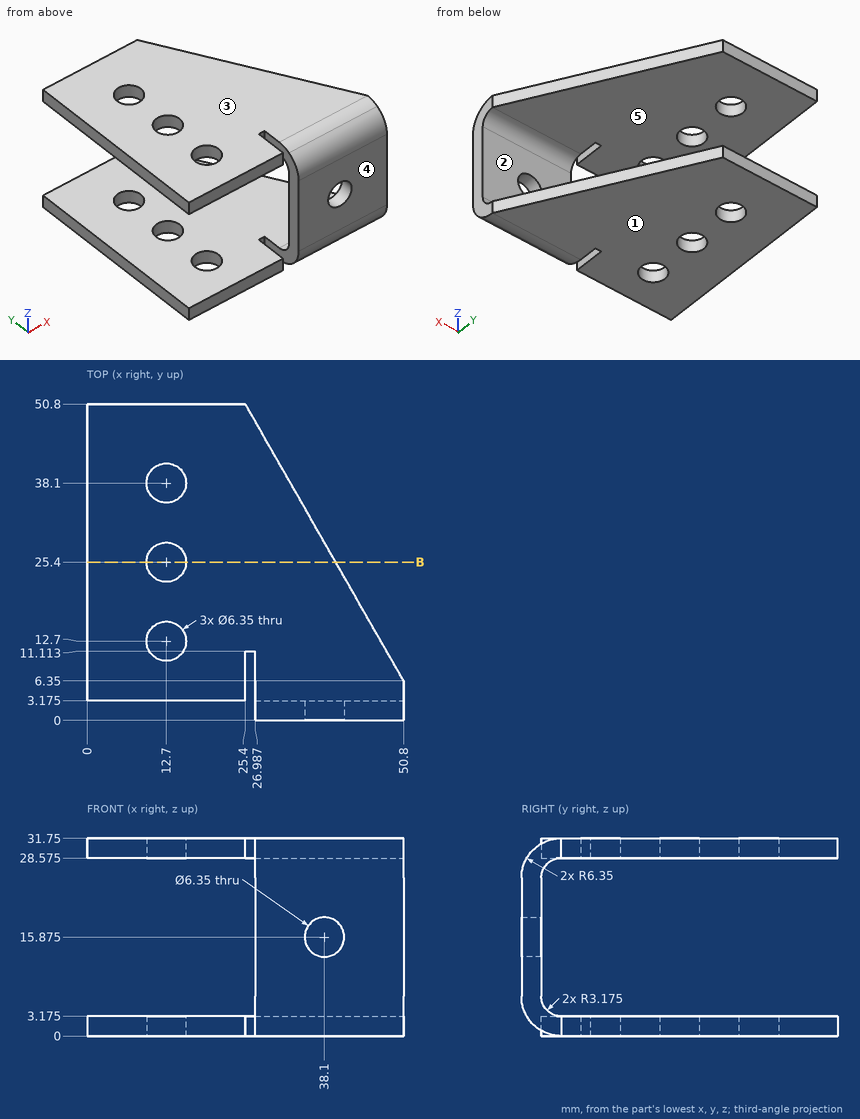
For this review, use the dimensioned drawing (mm, ordinates from the lowest corner) and the shaded views. A direction names the side the tool comes from. Coordinates: 2 decimals unless noted, no trailing zeros. Use a Markdown table: item, result. Add a question column.
Item 1: We need section B-B, the plane y = 25.4. Count the separate pieces of the cut face and the enclosed holes in it, and give its area (3 significant figures).
Item 2: Wall thickness on L1, parallel to Y at x = 12.7, z = 2.5 (1 decimal); L2, parallel to Y at x = 16, z = 3 (1 decimal); L3, parallel to Y at x = 12, z = 1 (1 decimal): over which ranges is each line inside the solid? List them lowest first. Write a range as from..to.
Item 3: Clearance check with flat-ended pins moving along their axes: P1, Ø1.3, axis at x = 26.5, z = 1.5, coming from the -Y side; P2, Ø5.5, axis at x = 12.7, y = 12.7, coming from the -Z side; P3, Ø1.3, axis at x = 26, z = 29.5, coming from the -Y side (1 decimal); P4, Ø1, axis at y = 9, z = 1.5, coming from the +X side. State where each tip first meets the part, or that it passes through.
Item 4: The part is to be moulded in two halves that separate along Z. For the marked faces 3, 4 and 5, say which applies: +Z half, -Z half, draft (parallel to the pull), parting line (faces both ways), or undercut.
Item 5: Machinability: for the marked faces 1 and 2, which of the approach directions +Z, -Z, +X, -X, +Y, -Y give a long, thin tool a straight path to every point of the face, cutting with its end or side? Answer none if there is none.
Numbers:
| question | item | result |
|---|---|---|
| 1 | separate pieces | 4 |
| 1 | enclosed holes | 0 |
| 1 | area | 213 mm^2 |
| 2 | L1 | y = 3.2..9.5, 15.9..22.2, 28.6..34.9, 41.3..50.8 |
| 2 | L2 | y = 3.2..50.8 |
| 2 | L3 | y = 3.2..9.6, 15.8..22.3, 28.5..35, 41.2..50.8 |
| 3 | P1 | stops at y = 1.79 |
| 3 | P2 | passes through |
| 3 | P3 | stops at y = 3.2 |
| 3 | P4 | stops at x = 49.57 |
| 4 | face 3 | +Z half |
| 4 | face 4 | draft |
| 4 | face 5 | undercut |
| 5 | face 1 | -Z, +X, -X, +Y, -Y |
| 5 | face 2 | +X, -X, +Y |
